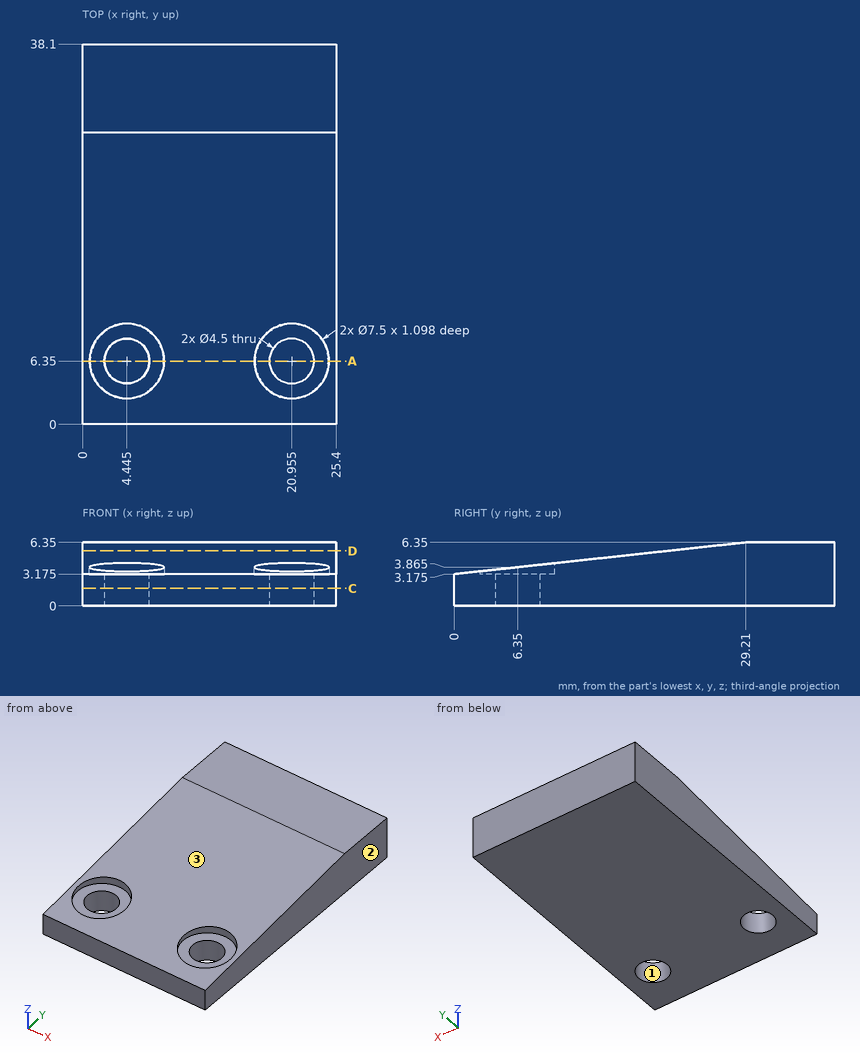
The figure shows three views and two pictorial views of one solid part (mm, origin at its lowest corner). Answer the questions. Coordinates: 2 decimals unless noted, no trailing zeros. Loops run counter-clockwise (first coordinate to the right, second up) from the corner with the lowest first, then second, coordinate; pieces in that order, holes last. Notation, with made-up numbers: (-15, 37.5) -> (18, 37.5) arc R20 cw to (18, 41.5) -> close; hole circle Ø10 at (-0.75, 1.5). An arc over 180 degrees is marked (long way). Write item = value, one per line. Start each with the question number.
1) Straight lines are drawn through the part: line 1 (Z direction, x = 22.5, y = 4.5) (3 decimals); line 2 (Y direction, x = 5, z = 2.5); line 3 (Z direction, x = 23.25, y = 12). For each, find the intervals that lie inside material, in ascending order. Write a range as from..to.
2) A cutting plane is placed at C-C (z = 1.75). Give the vertices of the cut face in (x, y) (3 decimals).
3) A cutting plane is placed at D-D (z = 5.5). Give the vertices of the cut face in (x, y), then the cut area to 3 significant figures.
4) A cutting plane is placed at A-A (y = 6.35). Give the vertices of the cut face in (x, z) (1 decimal).
5) Given pin 1 Ø6 at (x, y) = (3.5, 6) entering from +Z; pin 2 Ø7 at (x, y) = (4.445, 6.35) entering from +Z (3 decimals); pin 3 Ø8 at (x, y) = (20.5, 7) entering from +Z, each flat-ended and moving along its own axis, determine where each tip first touches the part or whether it passes through.
6) The mould has two halves that part along Y. Classify the marked faces 1, 2 and 3: released by +Y, released by -Y, zero draft, split by the parting line, or undercut.
Responses:
q1.line_1 = 0..3.175
q1.line_2 = 0..4.17, 8.53..38.1
q1.line_3 = 0..4.48
q2.outline = (0, 0) -> (25.4, 0) -> (25.4, 38.1) -> (0, 38.1) -> close; hole circle Ø4.5 at (4.445, 6.35); hole circle Ø4.5 at (20.955, 6.35)
q3.outline = (0, 21.39) -> (25.4, 21.39) -> (25.4, 38.1) -> (0, 38.1) -> close
q3.area = 424 mm²
q4.outline = (0, 0) -> (2.2, 0) -> (2.2, 3.2) -> (0.7, 3.2) -> (0.7, 3.9) -> (0, 3.9) -> close; (6.7, 0) -> (18.7, 0) -> (18.7, 3.2) -> (17.2, 3.2) -> (17.2, 3.9) -> (8.2, 3.9) -> (8.2, 3.2) -> (6.7, 3.2) -> close; (23.2, 0) -> (25.4, 0) -> (25.4, 3.9) -> (24.7, 3.9) -> (24.7, 3.2) -> (23.2, 3.2) -> close
q5.pin_1 = 3.98
q5.pin_2 = 3.175
q5.pin_3 = 4.37
q6.face_1 = undercut
q6.face_2 = zero draft
q6.face_3 = released by -Y
